Autodesk Inventor part; units mm, degrees
ref_plane "YZ Plane" through (0, 0, 0) normal (1, 0, 0) x (0, 1, 0)
ref_plane "XZ Plane" through (0, 0, 0) normal (0, 1, 0) x (-1, 0, 0)
ref_plane "XY Plane" through (0, 0, 0) normal (0, 0, 1) x (1, 0, 0)
sketch "Sketch1" plane through (0, 0, 0) normal (0, 1, 0) x (-1, 0, 0)
  circle A0 centre (0, 0) radius 2
  circle A1 centre (0, 0) radius 3
  circle A2 centre (0, 0) radius 5
  dimension "d0" = 4
  dimension "d1" = 6
  dimension "d2" = 10
extrude "Extrusion1" add sketch "Sketch1" along normal blind 0.2 contours A1 | A2
extrude "Extrusion2" add sketch "Sketch1" along normal blind 20 contours A1
fillet "Fillet1" radius 5 1 edges at (3, 0.2, 0)
extrude "Extrusion3" add sketch "Sketch1" along normal blind 15 contours A0
fillet "Fillet2" radius 2 1 edges at (2, 15, 0)
properties part number "ssd standoff"
Model file for the job. Use its own axes, mm. Round coordinates to 2 decimals unless told otherwise and drop trailing zeros. Loops run counter-clockwise (first coordinate to the right, second up) from the corner with the lowest first, then second, coordinate; pieces in that order, holes last. Notation, with made-up numbers: M 78,13.5 L 88,13.5 A6 ccw 88,23.5 Z; hole C 45,3.25 d7. An arc over 180 degrees is marked long. Put each result on its own line as item: value. Start each with the question number.
Item 1: Cut at C-C (y = 9). List the corners of the cut face in (x, z), then the cut area to 3 significant figures.
Item 2: Cut at D-D (y = 16.5). List the corners of the cut face in (x, z).
Item 3: Drop flat-ended pins along their axis: P1, Ø2, axis at y = 8, z = 0, coming from the -X side; P2, Ø6, axis at x = -3, y = 16, coming from the +Z side; P3, Ø1, axis at y = 8, z = 3, coming from the +X side. Give the stop position or say it passes through.
Item 4: Cut at A-A (z = 0). List the corners of the cut face in (x, y).
Item 5: Mould opens along Z. For faces 1 (the face through (-1, 20, -2)), 2 (the face through (0, 18, 2)), 3 (the face through (3, 12, 0)) say: released by +Z, released by -Z, zero draft, split by the parting line, or undercut.
Item 6: Drill centre lines: line 1 along Z through (x, y) = (0, 18.5); line 2 along X through (y, z) = (17.5, -1.75); line 3 along Z through (x, y) = (0.25, 11.75). Where is each one in solid material? Low to high.
Item 7: Cut at B-B (x = 0). List the corners of the cut face in (y, z), then the cut area to 3 significant figures.
Answer block:
1. outline: C 0,0 d6
1. area: 28.3 mm2
2. outline: C 0,0 d6; hole C 0,0 d3.87
3. P1: x = -3
3. P2: z = 3
3. P3: x = 1.66
4. outline: M -5,0 L 5,0 L 5,0.2 A5 cw 3,4.2 L 3,20 L 2,20 L 2,17 A2 cw -2,17 L -2,20 L -3,20 L -3,4.2 A5 cw -5,0.2 Z
5. face 1: zero draft
5. face 2: undercut
5. face 3: split by the parting line
6. line 1: -3 to -2, 2 to 3
6. line 2: -2.44 to -0.97, 0.97 to 2.44
6. line 3: -2.99 to 2.99
7. outline: M 0,-5 L 0.2,-5 A5 cw 4.2,-3 L 20,-3 L 20,-2 L 17,-2 A2 cw 17,2 L 20,2 L 20,3 L 4.2,3 A5 cw 0.2,5 L 0,5 Z
7. area: 107 mm2
